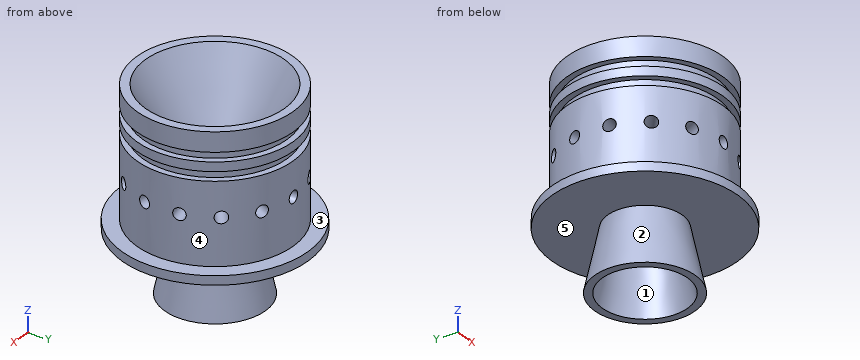
from build123d import *

# Parameters (mm, degrees)
MATRIZC1_COUNT = 14


with BuildPart() as part:
    # Croquis2 → Revolución1 (revolve)
    with BuildSketch(Plane(origin=(0, 0, 0), x_dir=(0, 0, -1), z_dir=(1, 0, 0))):
        with BuildLine():
            Line((0, 23.2509), (28.348346363, 6.883974596))
            ThreePointArc((28.348346363, 6.883974596), (28.589527318, 6.784074174), (28.848346363, 6.75))
            Line((28.848346363, 6.75), (30.3701887, 6.75))
            ThreePointArc((30.3701887, 6.75), (30.579245627, 6.760956209), (30.786012082, 6.793704799))
            Line((30.786012082, 6.793704799), (66.100354497, 14.3))
            Line((66.100354497, 14.3), (66.100354497, 16.855851487))
            Line((66.100354497, 16.855851487), (45.580397171, 12.494199912))
            Line((45.580397171, 12.494199912), (45.580397171, 26.0993))
            Line((45.580397171, 26.0993), (45.580397171, 31.1493))
            Line((45.580397171, 31.1493), (42.580397171, 31.1493))
            Line((42.580397171, 31.1493), (42.580397171, 26.1493))
            Line((42.580397171, 26.1493), (15.62, 26.1493))
            Line((15.62, 26.1493), (15.62, 24.0993))
            Line((15.62, 24.0993), (12.572, 24.0993))
            Line((12.572, 24.0993), (12.572, 26.1493))
            Line((12.572, 26.1493), (9.524, 26.1493))
            Line((9.524, 26.1493), (9.524, 24.0993))
            Line((9.524, 24.0993), (6.476, 24.0993))
            Line((6.476, 24.0993), (6.476, 26.1493))
            Line((6.476, 26.1493), (0, 26.1493))
            Line((0, 26.1493), (0, 23.2509))
        make_face()
    revolve(axis=Axis((0, 0, 14.017218159), (0, 0, -1)))

    # Croquis5 → Ø4.0mm Dowel Hole1 (revolve, cut)
    with BuildSketch(Plane(origin=(0, 26.1493, -27.080397171), x_dir=(0, 0, 1), z_dir=(1, 0, 0))):
        Polygon((0, 0), (0, 8.201721238), (2, 7), (2, 0), align=None)
    f_4_0mm_dowel_hole1 = revolve(axis=Axis((0, 32.4993, -27.080397171), (0, -1, 0)), mode=Mode.SUBTRACT)

    # MatrizC1: Ø4.0mm Dowel Hole1 ×14 about axis
    matrizc1_axis = Axis((0, 0, -15.62), (0, 0, 1))
    for i in range(1, MATRIZC1_COUNT):
        add(f_4_0mm_dowel_hole1.rotate(matrizc1_axis, i * 360 / MATRIZC1_COUNT), mode=Mode.SUBTRACT)


solid = part.part
Read the model definition and answer for the solid it produces. Units are mm, in the model's axes. Face numbers are marked on the shaded views. A direction names the side the tool comes from. Round coordinates to 2 decimals unless told otherwise and drop trailing zeros. Write each loop counter-clockwise with the first axis right and the second up, starting at its lowest first coordinate (ties: lowest second). Pieces come first, ordered by that corner, then holes.
1. Which of the six approach directions +Z, -Z, +X, -X, +Y, -Y give full straight-line access (tool end or side, diameter ignored) to the marked faces 4 and 5?
2. Determine the mould class of the marked faces 1, 2 and 3 for opening direction X: pulls with the +X half, pulls with the -X half, needs draft (parallel to the pull), parting line crosses it, or undercut.
3. Given pin 1 Ø8 at (y, z) = (-14.5, -22) entering from -X; pin 2 Ø4 at (x, z) = (6.5, -55.5) entering from +Y; pin 3 Ø3 at (y, z) = (-19.5, -26) entering from +X; pin 4 Ø15.5 at (x, y) = (-9, 10) entering from -Z, each flat-ended and moving along its own axis, determine where each tip first touches the part or whether it passes through.
4. The part is cut by section A-A, the plane z = -59. Determine the outline of the cut face in (x, y), then the cut area to 3 significant figures.
5. Straight lines are drawn through the part: L1, parallel to X at y = 0, z = -29.6; L2, parallel to X at y = 19, z = -27; L3, parallel to Y at x = 8.5, z = -27. For each, find the intervals that lie inside material, in ascending order.
Values:
1. face 4: +Z
1. face 5: none
2. face 1: undercut
2. face 2: parting line crosses it
2. face 3: needs draft
3. pin 1: stops at x = -23.95
3. pin 2: stops at y = 14.03
3. pin 3: stops at x = 18.97
3. pin 4: stops at z = -66.1
4. outline: circle Ø30.69 at (0, 0); hole circle Ø25.58 at (0, 0)
4. area: 226 mm2
5. L1: x = -26.15 to -6.75, 6.75 to 26.15
5. L2: x = -17.97 to -11.37, -6.93 to -1.75, 1.75 to 6.93, 11.37 to 17.97
5. L3: y = -24.73 to -22.26, -16.24 to 16.24, 22.26 to 24.73
